The listing builds one solid part. Answer for the finished solid, in the listing's coordinates (mm). A direction names the side the tool comes from. Coordinates: 2 decimals unless noted, no trailing zeros. Write each loop counter-clockwise with the first axis right and the second up, starting at its lowest first coordinate (ties: lowest second). Pieces come first, ordered by that corner, then holes.
from build123d import *

# Parameters (mm, degrees)
F0_R     = 6.35
F1_DEPTH = 12.7
F0_W     = 12.7
F0_H     = 38.1
F2_DEPTH = 25.4
F4_DEPTH = 12.7


with BuildPart() as f1:
    # F0 (on Top) → F1 (new body)
    with BuildSketch(Plane.XY):
        with BuildLine():
            Line((12.7, 38.1), (12.7, 0))
            Line((12.7, 0), (50.8, 0))
            ThreePointArc((50.8, 0), (69.85, 19.05), (50.8, 38.1))
            Line((50.8, 38.1), (12.7, 38.1))
        make_face()
        with Locations((50.8, 19.05)):
            Circle(F0_R, mode=Mode.SUBTRACT)
    extrude(amount=-F1_DEPTH)

    # F0 (on Top) → F2 (join)
    with BuildSketch(Plane.XY):
        with Locations((6.35, 19.05)):
            Rectangle(F0_W, F0_H)
    extrude(amount=-F2_DEPTH)

    # F3 (on face) → F4 (join)
    with BuildSketch(Plane(origin=(0, 38.1, 0), x_dir=(-1, 0, 0), z_dir=(0, 1, 0))):
        with BuildLine():
            Line((-25.4, 0), (0, 0))
            Line((0, 0), (0, 6.35))
            ThreePointArc((0, 6.35), (-12.7, 19.05), (-25.4, 6.35))
            ThreePointArc((-25.4, 6.35), (-27.127977, 1.985086), (-31.382129, 0))
            Line((-31.382129, 0), (-25.4, 0))
        make_face()
    extrude(amount=-F4_DEPTH)


solid = f1.part
1. Section C-C on x = 53 is taken. Give the vertices of the cut face in (y, z).
Results found:
outline: (0.13, -12.7) - (13.09, -12.7) - (13.09, 0) - (0.13, 0) - close; (25.01, -12.7) - (37.97, -12.7) - (37.97, 0) - (25.01, 0) - close
2. Section D-D on x = 40 is taken. Give the vertices of the cut face in (y, z), then the cut area to 3 significant figures.
Results found:
outline: (0, -12.7) - (38.1, -12.7) - (38.1, 0) - (0, 0) - close
area: 484 mm2
3. Find the intervals of material crossed by L1, parallel to Y at x = 50.8, z = -3.5; L2, parallel to X at y = 19, z = -3; L3, parallel to Z at x = 33, y = 4, in increasing order.
Results found:
L1: y = 0 to 12.7, 25.4 to 38.1
L2: x = 0 to 44.45, 57.15 to 69.85
L3: z = -12.7 to 0
4. Flat-ended cylindrical pins translate along their axes: P1, Ø9.5, axis at x = 14, z = 14, coming from the -Y side; P2, Ø1.5, axis at x = 52, y = 9, coming from the -Z side; P3, Ø4, axis at y = 10, z = -18.5, coming from the +X side. Find the tip coordinate at first contact, or state that the pin passes through.
Results found:
P1: stops at y = 25.4
P2: stops at z = -12.7
P3: stops at x = 12.7
5. Section B-B on z = -3.5 is taken. Give the vertices of the cut face in (x, y).
Results found:
outline: (0, 0) - (50.8, 0) arc R19.05 ccw to (50.8, 38.1) - (0, 38.1) - close; hole circle Ø12.7 at (50.8, 19.05)
6. A tool of negligible diameter and unlimited length cuts with its end or side. For faces 1 (the flat face through (34, 15, 0)), 2 (the flat face through (19, 0, -10)), 3 (the flat face through (41, 19, -12.7)), from which of +Z, -Z, +X, -X, +Y, -Y can it reach the whole face along a straight path? Write none if from no direction.
Results found:
face 1: +Z, +X, -Y
face 2: +Z, -Z, +X, -X, -Y
face 3: -Z, +X, +Y, -Y
7. Section A-A on y = 19.05 is taken. Give the vertices of the cut face in (x, z).
Results found:
outline: (0, -25.4) - (12.7, -25.4) - (12.7, -12.7) - (44.45, -12.7) - (44.45, 0) - (0, 0) - close; (57.15, -12.7) - (69.85, -12.7) - (69.85, 0) - (57.15, 0) - close
8. For a pull along Y with two mould halves and no side action, classify faces 4 (the flat face through (12.7, 19, -19)), 5 (the cylindrical face through (56.857, 20.957, -6.261)), 6 (the flat face through (12, 25.4, 10)) as pulls with the +Y half, pulls with the -Y half, needs draft (parallel to the pull), parting line crosses it, or undercut.
Results found:
face 4: needs draft
face 5: undercut
face 6: pulls with the -Y half
